from build123d import *
from build123d.topology import SkipClean

# Parameters (mm, degrees)
SKETCH1_W           = 60
SKETCH1_H           = 28
SKETCH1_R           = 4.25
BOSS_EXTRUDE1_DEPTH = 5
SKETCH2_W           = 20
SKETCH2_H           = 12.5
CUT_EXTRUDE1_DEPTH  = 35.583232932
SKETCH3_R           = 1.75
CUT_EXTRUDE2_DEPTH  = 30
CUT_EXTRUDE3_REACH  = 43.34
SKETCH4_R           = 1.75
FILLET1_R           = 5
FILLET2_R           = 2
SKETCH5_R           = 3.25
CUT_EXTRUDE4_DEPTH  = 4
SKETCH6_R           = 2.1
CUT_EXTRUDE5_DEPTH  = 2
SKETCH7_R           = 3
SKETCH7_R_2         = 1.75
BOSS_EXTRUDE2_DEPTH = 2
BOSS_EXTRUDE3_START = 2
SKETCH8_R           = 3
SKETCH8_R_2         = 1.75
BOSS_EXTRUDE3_DEPTH = 2
SKETCH9_R           = 2.1
CUT_EXTRUDE6_DEPTH  = 3
CHAMFER1_SIZE       = 0.5
CHAMFER2_SIZE       = 1


with BuildPart() as part:
    # Sketch1 → Boss-Extrude1 (new, symmetric)
    with BuildSketch(Plane.XY):
        Rectangle(SKETCH1_W, SKETCH1_H)
        with Locations((-22, -6)):
            Circle(SKETCH1_R, mode=Mode.SUBTRACT)
        with Locations((22, -6)):
            Circle(SKETCH1_R, mode=Mode.SUBTRACT)
    extrude(amount=BOSS_EXTRUDE1_DEPTH, both=True)

    # Sketch2 → Cut-Extrude1 (cut, through all)
    with BuildSketch(Plane(origin=(0, 0, -5), x_dir=(-1, 0, 0), z_dir=(0, 0, -1))):
        with Locations((0, 2.5)):
            Rectangle(SKETCH2_W, SKETCH2_H)
    extrude(amount=-CUT_EXTRUDE1_DEPTH, mode=Mode.SUBTRACT)

    # Sketch3 → Cut-Extrude2 (cut)
    with BuildSketch(Plane(origin=(0, 14, 0), x_dir=(1, 0, 0), z_dir=(0, 1, 0))):
        with Locations(Location((0, 0, 0), (0, 0, 270))):
            Circle(SKETCH3_R)
    extrude(amount=-CUT_EXTRUDE2_DEPTH, mode=Mode.SUBTRACT)

    # Sketch4 → Cut-Extrude3 (cut, up to next)
    with BuildSketch(Plane(origin=(0, -14, 0), x_dir=(1, 0, 0), z_dir=(0, 1, 0)), mode=Mode.PRIVATE) as cut_extrude3_sk1:
        with Locations(Location((-22, 0, 0), (0, 0, 90))):
            Circle(SKETCH4_R)
    cut_extrude3_tool1 = extrude(cut_extrude3_sk1.sketch, amount=CUT_EXTRUDE3_REACH, mode=Mode.PRIVATE) & part.part
    # Sketch4 → Cut-Extrude3 (cut, up to next)
    with BuildSketch(Plane(origin=(0, -14, 0), x_dir=(1, 0, 0), z_dir=(0, 1, 0)), mode=Mode.PRIVATE) as cut_extrude3_sk2:
        with Locations(Location((22, 0, 0), (0, 0, 90))):
            Circle(SKETCH4_R)
    cut_extrude3_tool2 = extrude(cut_extrude3_sk2.sketch, amount=CUT_EXTRUDE3_REACH, mode=Mode.PRIVATE) & part.part
    add(cut_extrude3_tool1.solids().sort_by_distance((-22, -14, 0))[0], mode=Mode.SUBTRACT)
    add(cut_extrude3_tool2.solids().sort_by_distance((22, -14, 0))[0], mode=Mode.SUBTRACT)

    # Fillet1
    fillet1_edges = [part.edges().sort_by_distance(p)[0] for p in [
        (-30, 14, 0),
        (30, 14, 0),
        (30, -14, 0),
        (-30, -14, 0),
    ]]
    fillet(fillet1_edges, radius=FILLET1_R)

    # Fillet2
    fillet2_edges = [part.edges().sort_by_distance(p)[0] for p in [
        (-10, 8.75, 0),
        (-10, -3.75, 0),
        (10, -3.75, 0),
        (10, 8.75, 0),
    ]]
    fillet(fillet2_edges, radius=FILLET2_R)

    # Sketch5 → Cut-Extrude4 (cut)
    with BuildSketch(Plane.XZ.offset(14)):
        with Locations(Location((0, 0, 0), (0, 0, 270))):
            Circle(SKETCH5_R)
    extrude(amount=-CUT_EXTRUDE4_DEPTH, mode=Mode.SUBTRACT)

    # Sketch6 → Cut-Extrude5 (cut)
    with BuildSketch(Plane(origin=(0, -14, 0), x_dir=(1, 0, 0), z_dir=(0, 1, 0))):
        with Locations(Location((-22, 0, 0), (0, 0, 270))):
            Circle(SKETCH6_R)
        with Locations(Location((22, 0, 0), (0, 0, 270))):
            Circle(SKETCH6_R)
    extrude(amount=CUT_EXTRUDE5_DEPTH, mode=Mode.SUBTRACT)

    # Sketch7 → Boss-Extrude2 (add)
    with SkipClean():  # the faces are left unmerged after this step: merging them gives an invalid solid
        with BuildSketch(Plane.XZ.offset(-8.75)):
            with Locations(Location((0, 0, 0), (0, 0, 180))):
                Circle(SKETCH7_R)
            Circle(SKETCH7_R_2, mode=Mode.SUBTRACT)
        extrude(amount=BOSS_EXTRUDE2_DEPTH)

    # Sketch8 → Boss-Extrude3 (add)
    with SkipClean():  # the faces are left unmerged after this step: merging them gives an invalid solid
        with BuildSketch(Plane(origin=(0, -3.75, 0), x_dir=(1, 0, 0), z_dir=(0, 1, 0)).offset(BOSS_EXTRUDE3_START)):
            with Locations(Location((0, 0, 0), (0, 0, 180))):
                Circle(SKETCH8_R)
            with Locations(Location((0, 0, 0), (0, 0, 180))):
                Circle(SKETCH8_R_2, mode=Mode.SUBTRACT)
        extrude(amount=-BOSS_EXTRUDE3_DEPTH)

    # Sketch9 → Cut-Extrude6 (cut)
    with SkipClean():  # the faces are left unmerged after this step: merging them gives an invalid solid
        with BuildSketch(Plane(origin=(0, 14, 0), x_dir=(1, 0, 0), z_dir=(0, 1, 0))):
            with Locations(Location((0, 0, 0), (0, 0, 270))):
                Circle(SKETCH9_R)
        extrude(amount=-CUT_EXTRUDE6_DEPTH, mode=Mode.SUBTRACT)

    # Chamfer1
    # the kernel refuses this chamfer: 0.5 mm, written as the material it takes off along each edge
    with BuildSketch(Plane(origin=(22, -12, 0), x_dir=(0, 0, -1), z_dir=(-1, 0, 0))) as chamfer1_piece_1_section:
        Polygon((1.75, -CHAMFER1_SIZE), (1.75 + CHAMFER1_SIZE, 0), (1.75, 0), align=None)
    chamfer1_piece_1 = revolve(axis=Axis((22, -12, 0), (0, -1, 0)), mode=Mode.PRIVATE)
    chamfer1_piece_1 = chamfer1_piece_1 & Plane(origin=(22, -11.675956313, 0), x_dir=(0, 0, 1), z_dir=(0, -1, 0)) * Cylinder(2.1, 9, mode=Mode.PRIVATE)
    add(chamfer1_piece_1, mode=Mode.SUBTRACT)
    with BuildSketch(Plane(origin=(-22, -12, 0), x_dir=(0, 0, -1), z_dir=(-1, 0, 0))) as chamfer1_piece_2_section:
        Polygon((1.75, -CHAMFER1_SIZE), (1.75 + CHAMFER1_SIZE, 0), (1.75, 0), align=None)
    chamfer1_piece_2 = revolve(axis=Axis((-22, -12, 0), (0, -1, 0)), mode=Mode.PRIVATE)
    chamfer1_piece_2 = chamfer1_piece_2 & Plane(origin=(-22, -11.675956313, 0), x_dir=(0, 0, 1), z_dir=(0, -1, 0)) * Cylinder(2.1, 9, mode=Mode.PRIVATE)
    add(chamfer1_piece_2, mode=Mode.SUBTRACT)
    with BuildSketch(Plane(origin=(0, 11, 0), x_dir=(0, 0, 1), z_dir=(-1, 0, 0))) as chamfer1_piece_3_section:
        Polygon((1.75 + CHAMFER1_SIZE, 0), (1.75, -CHAMFER1_SIZE), (1.75, 0), align=None)
    chamfer1_piece_3 = revolve(axis=Axis((0, 11, 0), (0, 1, 0)), mode=Mode.PRIVATE)
    chamfer1_piece_3 = chamfer1_piece_3 & Plane(origin=(0, 10.675956313, 0), x_dir=(0, 0, 1), z_dir=(0, 1, 0)) * Cylinder(2.1, 9, mode=Mode.PRIVATE)
    add(chamfer1_piece_3, mode=Mode.SUBTRACT)

    # Chamfer2
    chamfer2_edges = [part.edges().sort_by_distance(p)[0] for p in [
        (3, 8.75, 0),
        (3, -3.75, 0),
    ]]
    chamfer(chamfer2_edges, length=CHAMFER2_SIZE)


solid = part.part
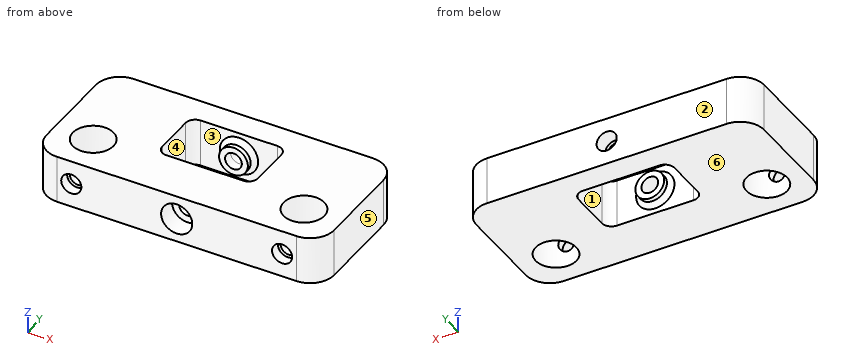
Read the model definition and answer for the solid it produces. Units are mm, in the model's axes. Face numbers are marked on the shaded views. A direction names the side the tool comes from. Round coordinates to 2 decimals unless told otherwise and drop trailing zeros. Loops run counter-clockwise (first coordinate to the right, second up) from the corner with the lowest first, then second, coordinate; pieces in that order, holes last.
Q1. Section A-A on y = -6 is taken. Write down the section's boundary in (x, z).
Q2. Section C-C on x = 0 is taken. Give the number of separate pieces and of enclosed holes in the cut face, and give its area (3 significant figures).
Q3. Which of the six approach directions +Z, -Z, +X, -X, +Y, -Y give full straight-line access (tool end or side, diameter ignored) to the marked faces 1, 2 and 3?
Q4. Determine the mould class of the marked faces 4, 5 and 6 for opening direction X: released by +X, released by -X, zero draft, split by the parting line, or undercut.
Q5. Each of these flat-tipped pins is pushed along its axis until it touches: pin 1 (5 mm diameter, centred on x = 0, z = 0, fed in from -Y); pin 2 (4 mm diameter, centred on x = 0, z = 0, fed in from +Y). Where does it stop, or does it pass through?
Q6. Consider probe 1 along X at (y, z) = (-6.25, 0); probe 2 along Y at (x, z) = (-25, -4); probe 3 along Y at (x, z) = (7, -0.25). Determine where each line is inside the solid, lowest interval first.
Q7. Section B-B on x = -7 is taken. Write down the section's boundary in (y, z), and give its area (3 significant figures).
Output:
1. outline: (-30, -5) - (-26.25, -5) - (-26.25, 5) - (-30, 5) - close; (-17.75, -5) - (17.75, -5) - (17.75, 5) - (-17.75, 5) - close; (26.25, -5) - (30, -5) - (30, 5) - (26.25, 5) - close; hole circle Ø3.5 at (0, 0)
2. separate pieces: 4
2. enclosed holes: 0
2. area: 98.4 mm2
3. face 1: +Z, -Z
3. face 2: +Z, -Z, +X, -X, +Y
3. face 3: none
4. face 4: undercut
4. face 5: released by +X
4. face 6: zero draft
5. pin 1: stops at y = -10
5. pin 2: stops at y = 10.75
6. probe 1: x = -30 to -26.24, -17.76 to -1.75, 1.75 to 17.76, 26.24 to 30
6. probe 2: y = -14 to -9.01, -2.99 to 14
6. probe 3: y = -14 to -3.75, 8.75 to 14
7. outline: (-14, -5) - (-3.75, -5) - (-3.75, 5) - (-14, 5) - close; (8.75, -5) - (14, -5) - (14, 5) - (8.75, 5) - close
7. area: 155 mm2
